Read the model definition and answer for the solid it produces. Units are mm, in the model's axes. A direction names the side the tool comes from. Coordinates: 2 decimals unless noted, no trailing zeros. Order: outer loops, then holes, each group sorted by start corner. A loop starts at its lowest first (then second) coordinate and runs counter-clockwise, first axis right, second up. Notation, with made-up numbers: M 44.25,-35 L 65.25,-35 A18 ccw 65.25,-11 Z; hole C -3.5,5.5 d6. An arc over 180 degrees is marked long. Use a Markdown table: item, result. Add a question column.
1) For faces 1 (the face through (3.091, 0.987, -3.135)), 2 (the face through (-16, 0.2, 0)), 3 (the face through (-20, -0.4, 0)), 4 (the face through (5, -2, 0)), determine the directions among +Z, -Z, +X, -X, +Y, -Y from which every point of the face is accessible in a straight line to the end or side of a thin tool.
2) Find section D-D on x = -18. Write down the section's boundary in (y, z).
3) Find section B-B on x = -11.5. Write down the section's boundary in (y, z), plus the area to 3 significant figures.
4) Find section C-C on y = 3.25. Count the separate pieces of the cut face and the enclosed holes in it, plus the area to 3 significant figures.
5) Find the intervals of material crossed by probe 1 along Y at (x, z) = (1.5, 0); probe 2 along Z at (x, y) = (-1.5, 1.75); probe 3 along Y at (x, z) = (3, 0), in increasing order. Write a range as [from, to].
6) Each of these flat-tipped pins is pushed along its axis until it touches: pin 1 Ø1 at (x, z) = (-1, 0.5) entering from +Y; pin 2 Ø0.7 at (x, z) = (-13, 0) entering from +Y; pin 3 Ø2 at (x, z) = (-17, 0.5) entering from -Y; pin 4 Ø3 at (y, z) = (0.5, 3) entering from -X. Where does it stop, or does it pass through?
7) The mould has two halves that part along X. Classify faces 5 (the face through (15, 2, -1)), 6 (the face through (8.091, 0.145, 3.283)), 7 (the face through (-16, -0.2, 0)): released by +X, released by -X, zero draft, split by the parting line, or undercut.
8) Find section A-A on z = 0. Write down the section's boundary in (x, y), plus the area to 3 significant figures.
from build123d import *

# Parameters (mm, degrees)
SKETCH1_R           = 4
BOSS_EXTRUDE1_DEPTH = 5
BOSS_EXTRUDE1_TAPER = 13
SKETCH2_R           = 4
BOSS_EXTRUDE2_DEPTH = 5
BOSS_EXTRUDE2_TAPER = 13
SKETCH3_R           = 4
BOSS_EXTRUDE3_DEPTH = 5
BOSS_EXTRUDE3_TAPER = 13
SKETCH4_R           = 2.85
BOSS_EXTRUDE4_DEPTH = 2
SKETCH5_R           = 2.85
BOSS_EXTRUDE5_DEPTH = 3
BOSS_EXTRUDE5_DRAFT = -35
SKETCH6_R           = 4.950622615
BOSS_EXTRUDE6_DEPTH = 15
BOSS_EXTRUDE6_TAPER = 12
SKETCH9_R           = 2
CUT_EXTRUDE1_DEPTH  = 20
SKETCH12_W          = 2.479913688
SKETCH12_H          = 0.4
CUT_EXTRUDE10_DEPTH = 10
SKETCH14_R          = 2
CUT_EXTRUDE11_DEPTH = 10
CUT_EXTRUDE11_DRAFT = -11.2


with BuildPart() as part:
    # Sketch1 → Boss-Extrude1 (new body)
    with BuildSketch(Plane(origin=(0, 0, 0), x_dir=(0, 0, -1), z_dir=(1, 0, 0))):
        Circle(SKETCH1_R)
    extrude(amount=BOSS_EXTRUDE1_DEPTH, taper=BOSS_EXTRUDE1_TAPER)

    # Sketch2 → Boss-Extrude2 (add)
    with BuildSketch(Plane(origin=(5, 0, 0), x_dir=(0, 0, -1), z_dir=(1, 0, 0))):
        Circle(SKETCH2_R)
    extrude(amount=BOSS_EXTRUDE2_DEPTH, taper=BOSS_EXTRUDE2_TAPER)

    # Sketch3 → Boss-Extrude3 (add)
    with BuildSketch(Plane(origin=(10, 0, 0), x_dir=(0, 0, -1), z_dir=(1, 0, 0))):
        Circle(SKETCH3_R)
    extrude(amount=BOSS_EXTRUDE3_DEPTH, taper=BOSS_EXTRUDE3_TAPER)

    # Sketch4 → Boss-Extrude4 (add)
    with BuildSketch(Plane.ZY):
        Circle(SKETCH4_R)
    extrude(amount=BOSS_EXTRUDE4_DEPTH)


with BuildPart() as boss_extrude5_tool:
    # Sketch5 → Boss-Extrude5 (with draft: the straight prism first)
    with BuildSketch(Plane.ZY.offset(2)):
        Circle(SKETCH5_R)
    extrude(amount=BOSS_EXTRUDE5_DEPTH)
    # Boss-Extrude5: the draft: its side faces are tilted about the plane it starts from
    boss_extrude5_sides = [boss_extrude5_tool.faces().sort_by_distance(p)[0] for p in [
        (-3.5, 0, -2.85),
    ]]
    draft(boss_extrude5_sides, Plane.ZY.offset(2), BOSS_EXTRUDE5_DRAFT)


with BuildPart() as part_1:
    add(part.part)

    # Boss-Extrude5: add boss_extrude5_tool
    add(boss_extrude5_tool.part)

    # Sketch6 → Boss-Extrude6 (add)
    with BuildSketch(Plane.ZY.offset(5)):
        Circle(SKETCH6_R)
    extrude(amount=BOSS_EXTRUDE6_DEPTH, taper=BOSS_EXTRUDE6_TAPER)

    # Sketch9 → Cut-Extrude1 (cut)
    with BuildSketch(Plane(origin=(15, 0, 0), x_dir=(0, 0, -1), z_dir=(1, 0, 0))):
        Circle(SKETCH9_R)
    extrude(amount=-CUT_EXTRUDE1_DEPTH, mode=Mode.SUBTRACT)

    # Sketch12 → Cut-Extrude10 (cut)
    with BuildSketch(Plane.ZY.offset(20)):
        Rectangle(SKETCH12_W, SKETCH12_H)
    extrude(amount=-CUT_EXTRUDE10_DEPTH, mode=Mode.SUBTRACT)


with BuildPart() as cut_extrude11_tool:
    # Sketch14 → Cut-Extrude11 (with draft: the straight prism first)
    with BuildSketch(Plane(origin=(-5, 0, 0), x_dir=(0, 0, -1), z_dir=(1, 0, 0))):
        Circle(SKETCH14_R)
    extrude(amount=-CUT_EXTRUDE11_DEPTH)
    # Cut-Extrude11: the draft: its side faces are tilted about the plane it starts from
    cut_extrude11_sides = [cut_extrude11_tool.faces().sort_by_distance(p)[0] for p in [
        (-10, 0, 2),
    ]]
    draft(cut_extrude11_sides, Plane(origin=(-5, 0, 0), x_dir=(0, 0, -1), z_dir=(1, 0, 0)), CUT_EXTRUDE11_DRAFT)


with BuildPart() as part_2:
    add(part_1.part)

    # Cut-Extrude11: cut by cut_extrude11_tool
    add(cut_extrude11_tool.part, mode=Mode.SUBTRACT)


solid = part_2.part
Check result:
| question | item | result |
|---|---|---|
| 1 | face 1 | none |
| 1 | face 2 | -X |
| 1 | face 3 | +Z, -Z, -X, +Y, -Y |
| 1 | face 4 | +X |
| 2 | outline | C 0,0 d4.37; hole M -0.2,-1.24 L 0.2,-1.24 L 0.2,1.24 L -0.2,1.24 Z |
| 3 | outline | C 0,0 d7.14; hole M -0.2,-1.24 L 0.2,-1.24 L 0.2,-0.68 A0.71 ccw 0.2,0.68 L 0.2,1.24 L -0.2,1.24 L -0.2,0.68 A0.71 ccw -0.2,-0.68 Z |
| 3 | area | 38.0 mm2 |
| 4 | separate pieces | 4 |
| 4 | enclosed holes | 0 |
| 4 | area | 79.4 mm2 |
| 5 | probe 1 | y = [-3.65, -2], [2, 3.65] |
| 5 | probe 2 | z = [-2.25, -0.97], [0.97, 2.25] |
| 5 | probe 3 | y = [-3.31, -2], [2, 3.31] |
| 6 | pin 1 | stops at y = 2.85 |
| 6 | pin 2 | stops at y = 3.32 |
| 6 | pin 3 | stops at y = -2.6 |
| 6 | pin 4 | stops at x = -20 |
| 7 | face 5 | released by +X |
| 7 | face 6 | undercut |
| 7 | face 7 | zero draft |
| 8 | outline | M -20,-1.76 L -5,-4.95 L -2,-2.85 L 0,-2.85 L 0,-4 L 5,-2.85 L 5,-4 L 10,-2.85 L 10,-4 L 15,-2.85 L 15,-2 L -5,-2 L -14.09,-0.2 L -20,-0.2 Z; M -20,0.2 L -14.09,0.2 L -5,2 L 15,2 L 15,2.85 L 10,4 L 10,2.85 L 5,4 L 5,2.85 L 0,4 L 0,2.85 L -2,2.85 L -5,4.95 L -20,1.76 Z |
| 8 | area | 136 mm2 |
